Geometry: final body of the model. Coordinates: model frame, mm. A direction names the side the tool comes from. Give positions to 0.01 mm unless a question says otherwise; leave off trailing zeros.
Q1. Reachability of faces 1 (the flat face through (-18.2, -4, -1)), 2 (the flat face through (13.866, 9.113, -0.7)), 3 (the flat face through (-6.134, -9.113, -0.7)), 4 (the flat face through (19.113, -3.866, -0.7)) from +Z, -Z, +X, -X, +Y, -Y: full face, straight path, thin tool, end or side. Return the list, or none.
Q2. Section A-A (z = 26). State how many separate pieces and enclosed holes the cut face has, plus the area to 3 significant figures.
Q3. Mould query, pull axis Y, two halves, no side actions, for faces 5 (the flat face through (6.134, -9.113, -0.7)), 6 (the flat face through (-2.383, 7, -1)), 7 (the flat face through (0, 10, -1)). Classes: +Y half, -Y half, draft (parallel to the pull), parting line (faces both ways), or undercut.
Q4. Line query: line 1 (X direction, y = -7, z = -27.5); line 2 (Y direction, x = 10, z = 22); line 3 (X direction, y = 1.75, z = 20). Output: solid intervals per line, ascending.
Q5. Pin query (flat end, axial travel): pin 1 Ø0.7 at (x, z) = (5.5, -23.5) entering from +Y; pin 2 Ø2.5 at (x, z) = (8.5, 2) entering from -Y; pin 3 Ø0.7 at (y, z) = (-3.5, -23) entering from +X; pin 4 Ø0.7 at (x, z) = (-6.5, 17) entering from -Y. Return the tip coordinate at first contact, or that it passes through.
Autodesk Inventor part; units mm, degrees
ref_plane "YZ Plane" through (0, 0, 0) normal (1, 0, 0) x (0, 1, 0)
ref_plane "XZ Plane" through (0, 0, 0) normal (0, 1, 0) x (-1, 0, 0)
ref_plane "XY Plane" through (0, 0, 0) normal (0, 0, 1) x (1, 0, 0)
sketch "Sketch1" plane through (0, 0, 0) normal (0, 0, 1) x (1, 0, 0)
  line L0 (4.5, 8.2) -> (4.5, 6.5562)
  line L1 (6.9, 8.2) -> (4.5, 8.2)
  line L2 (5.3896, 10) -> (6.9, 8.2)
  line L3 (-5.3896, 10) -> (5.3896, 10)
  line L4 (-5.3896, 10) -> (-6.9, 8.2)
  line L5 (-6.9, 8.2) -> (-4.5, 8.2)
  line L6 (-4.5, 8.2) -> (-4.5, 6.5562)
  line L7 (-4.5, 6.5562) -> (-7.1607, 3.9)
  line L8 (-9.4804, 3.8998) -> (-7.1607, 3.9)
  line L9 (-9.4804, 3.8998) -> (-10, 3.5998)
  line L10 (-10.5196, 3.8998) -> (-10, 3.5998)
  line L11 (-12.8393, 3.9) -> (-10.5196, 3.8998)
  line L12 (-15.5, 6.5562) -> (-12.8393, 3.9)
  line L13 (-15.5, 8.2) -> (-15.5, 6.5562)
  line L14 (-13.1, 8.2) -> (-15.5, 8.2)
  line L15 (-14.6104, 10) -> (-13.1, 8.2)
  line L16 (-20, 10) -> (-14.6104, 10)
  line L17 (-20, 10) -> (-20, 4.6104)
  line L18 (-20, 4.6104) -> (-18.2, 3.1)
  line L19 (-18.2, 3.1) -> (-18.2, 5.5)
  line L20 (-16.5562, 5.5) -> (-18.2, 5.5)
  line L21 (-16.5562, 5.5) -> (-13.9, 2.8393)
  line L22 (-13.9, 0.5196) -> (-13.9, 2.8393)
  line L23 (-13.9, 0.5196) -> (-13.6, 0)
  line L24 (-13.6, 0) -> (-13.9, -0.5196)
  line L25 (-13.9, -2.8393) -> (-13.9, -0.5196)
  line L26 (-16.5562, -5.5) -> (-13.9, -2.8393)
  line L27 (-16.5562, -5.5) -> (-18.2, -5.5)
  line L28 (-18.2, -3.1) -> (-18.2, -5.5)
  line L29 (-20, -4.6104) -> (-18.2, -3.1)
  line L30 (-20, -10) -> (-20, -4.6104)
  line L31 (-20, -10) -> (-14.6104, -10)
  line L32 (-14.6104, -10) -> (-13.1, -8.2)
  line L33 (-13.1, -8.2) -> (-15.5, -8.2)
  line L34 (-15.5, -8.2) -> (-15.5, -6.5562)
  line L35 (-15.5, -6.5562) -> (-12.8393, -3.9)
  line L36 (-12.8393, -3.9) -> (-10.5196, -3.9002)
  line L37 (-10.5196, -3.9002) -> (-10, -3.6002)
  line L38 (-9.4804, -3.9002) -> (-10, -3.6002)
  line L39 (-9.4804, -3.9002) -> (-7.1604, -3.9002)
  line L40 (-4.5, -6.5562) -> (-7.1604, -3.9002)
  line L41 (-4.5, -8.2) -> (-4.5, -6.5562)
  line L42 (-6.9, -8.2) -> (-4.5, -8.2)
  line L43 (-5.3896, -10) -> (-6.9, -8.2)
  line L44 (-5.3896, -10) -> (5.3896, -10)
  line L45 (5.3896, -10) -> (6.9, -8.2)
  line L46 (6.9, -8.2) -> (4.5, -8.2)
  line L47 (4.5, -8.2) -> (4.5, -6.5562)
  line L48 (4.5, -6.5562) -> (7.1607, -3.9)
  line L49 (9.4808, -3.9) -> (7.1607, -3.9)
  line L50 (9.4808, -3.9) -> (10, -3.6002)
  line L51 (10.5192, -3.9) -> (10, -3.6002)
  line L52 (12.8393, -3.9) -> (10.5192, -3.9)
  line L53 (15.5, -6.5562) -> (12.8393, -3.9)
  line L54 (15.5, -8.2) -> (15.5, -6.5562)
  line L55 (13.1, -8.2) -> (15.5, -8.2)
  line L56 (14.6104, -10) -> (13.1, -8.2)
  line L57 (20, -10) -> (14.6104, -10)
  line L58 (20, -10) -> (20, -4.6104)
  line L59 (20, -4.6104) -> (18.2, -3.1)
  line L60 (18.2, -3.1) -> (18.2, -5.5)
  line L61 (16.5562, -5.5) -> (18.2, -5.5)
  line L62 (16.5562, -5.5) -> (13.9, -2.8393)
  line L63 (13.9, -2.8393) -> (13.9, -0.5196)
  line L64 (13.6, 0) -> (13.9, -0.5196)
  line L65 (13.9, 0.5196) -> (13.6, 0)
  line L66 (13.9, 0.5196) -> (13.9, 2.8393)
  line L67 (16.5562, 5.5) -> (13.9, 2.8393)
  line L68 (16.5562, 5.5) -> (18.2, 5.5)
  line L69 (18.2, 3.1) -> (18.2, 5.5)
  line L70 (20, 4.6104) -> (18.2, 3.1)
  line L71 (20, 10) -> (20, 4.6104)
  line L72 (20, 10) -> (14.6104, 10)
  line L73 (14.6104, 10) -> (13.1, 8.2)
  line L74 (13.1, 8.2) -> (15.5, 8.2)
  line L75 (15.5, 8.2) -> (15.5, 6.5562)
  line L76 (15.5, 6.5562) -> (12.8481, 3.8998)
  line L77 (10.5196, 3.8998) -> (12.8481, 3.8998)
  line L78 (10.5196, 3.8998) -> (10, 3.5998)
  line L79 (9.4804, 3.8998) -> (10, 3.5998)
  line L80 (7.1519, 3.8998) -> (9.4804, 3.8998)
  line L81 (4.5, 6.5562) -> (7.1519, 3.8998)
  circle A0 centre (-10, 0) radius 2
  circle A1 centre (10, 0) radius 2
  line L82 (6.1, 2.8393) -> (2.3832, 6.5562)
  line L83 (6.1, 2.8393) -> (6.1, -2.8393)
  line L84 (6.1, -2.8393) -> (2.3769, -6.5562)
  line L85 (2.3769, -6.5562) -> (2.3769, -8.2)
  line L86 (-2.3769, -8.2) -> (2.3769, -8.2)
  line L87 (-2.3769, -6.5562) -> (-2.3769, -8.2)
  line L88 (-6.1, -2.8393) -> (-2.3769, -6.5562)
  line L89 (-6.1, 2.8393) -> (-6.1, -2.8393)
  line L90 (-6.1, 2.8393) -> (-2.3832, 6.5562)
  line L91 (-2.3832, 6.5562) -> (-2.3832, 8.2)
  line L92 (-2.3832, 8.2) -> (2.3832, 8.2)
  line L93 (2.3832, 6.5562) -> (2.3832, 8.2)
  point P0 (0, 0)
  point P1 (0, 0)
extrude "Extrusion1" add sketch "Sketch1" along normal mid plane 100
properties part number "vslot_2040_100mm"
Computed:
1. face 1: +Z, -Z
1. face 2: +Z, -Z, +Y
1. face 3: +Z, -Z, -Y
1. face 4: +Z, -Z, +X
2. separate pieces: 1
2. enclosed holes: 3
2. area: 301 mm2
3. face 5: -Y half
3. face 6: undercut
3. face 7: +Y half
4. line 1: x = -20 to -15.5, -4.5 to -2.38, 2.38 to 4.5, 15.5 to 20
4. line 2: y = -3.6 to -2, 2 to 3.6
4. line 3: x = -13.9 to -10.97, -9.03 to -6.1, 6.1 to 9.03, 10.97 to 13.9
5. pin 1: stops at y = 10
5. pin 2: stops at y = -3.9
5. pin 3: stops at x = 19.09
5. pin 4: stops at y = -9.09
